Autodesk Inventor part; units mm, degrees
ref_plane "YZ Plane" through (0, 0, 0) normal (1, 0, 0) x (0, 1, 0)
ref_plane "XZ Plane" through (0, 0, 0) normal (0, 1, 0) x (-1, 0, 0)
ref_plane "XY Plane" through (0, 0, 0) normal (0, 0, 1) x (1, 0, 0)
sketch "Boceto1" plane through (0, 0, 0) normal (0, 0, 1) x (1, 0, 0)
  circle A0 centre (0, 0) radius 4
  circle A1 centre (0, 0) radius 1.5
  line L0 (0, -1) -> (1.5, -1)
  line L1 (1.5, -1) -> (-2.7531, -1)
  point P0 (1, -1.118)
  point P1 (1, 1.118)
  point P2 (-1.118, -1)
  point P3 (1.118, -1)
  dimension "d0" = 8
extrude "Extrusión1" add sketch "Boceto1" along normal blind 8 contours A0 | L1 L0 A1 picked at (-0.6553, -1.0791)
sketch "Boceto2" plane through (0, 0, 8) normal (0, 0, 1) x (1, 0, 0)
  circle A0 centre (0, 0) radius 8
  dimension "d3" = 16
extrude "Extrusión2" add sketch "Boceto2" along normal blind 10
sketch "Boceto3" plane through (0, 0, 18) normal (0, 0, 1) x (1, 0, 0)
  circle A0 centre (0, 0) radius 8
hole "Agujero1" at (0, 0, 18) direction (0, 0, -1) diameter 8 depth 8
sketch "Boceto5" plane through (0, 0, 0) normal (0, 1, 0) x (-1, 0, 0)
  line L0 (0, 0) -> (0, 4)
  circle A0 centre (0, 4) radius 1
  line L1 (0, 4) -> (0, 8)
  line L2 (0, 8) -> (0, 13)
  circle A1 centre (0, 13) radius 1.5
  dimension "d20" = 4
  dimension "d21" = 2
  dimension "d29" = 5
  dimension "d30" = 3
hole "Agujero3" at (0, 0, 4) direction (0, -1, 0) diameter 2 end through all
sketch "Boceto6" plane through (0, 0, 0) normal (0, 1, 0) x (-1, 0, 0)
  line L0 (0, 0) -> (0, 13)
  circle A0 centre (0, 13) radius 1.5
  dimension "d31" = 13
  dimension "d32" = 3
hole "Agujero4" at (0, 0, 13) direction (0, -1, 0) diameter 3 end through all
ref_plane "Plano de trabajo2" through (0, 0, 7) normal (0, 0, 1) x (-1, 0, 0)
sketch "Boceto7" plane through (0, 0, 7) normal (0, 0, 1) x (-1, 0, 0)
  circle A0 centre (0, 0) radius 17.5
  dimension "d42" = 35
extrude "Extrusión3" add sketch "Boceto7" along normal mid plane 1.5
sketch "Boceto8" plane through (0, 0, 7.75) normal (0, 0, 1) x (1, 0, 0)
  circle A0 centre (0, 0) radius 8
  circle A1 centre (0, 0) radius 17.5
  arc A2 (8.6603, -5) -> (10, 0) centre (0, 0) ccw
  arc A3 (14.2894, -8.25) -> (16.5, 0) centre (0, 0) ccw
  line L0 (10, 0) -> (16.5, 0)
  line L1 (0, 0) -> (16.5, 0) construction
  line L2 (8.6603, -5) -> (14.2894, -8.25)
  arc A4 (8.6603, 5) -> (5, 8.6603) centre (0, 0) ccw
  line L3 (8.6603, 5) -> (14.2894, 8.25)
  arc A5 (14.2894, 8.25) -> (8.25, 14.2894) centre (0, 0) ccw
  line L4 (5, 8.6603) -> (8.25, 14.2894)
  arc A6 (0, 10) -> (-5, 8.6603) centre (0, 0) ccw
  line L5 (0, 10) -> (0, 16.5)
  arc A7 (0, 16.5) -> (-8.25, 14.2894) centre (0, 0) ccw
  line L6 (-5, 8.6603) -> (-8.25, 14.2894)
  arc A8 (-8.6603, 5) -> (-10, 0) centre (0, 0) ccw
  line L7 (-8.6603, 5) -> (-14.2894, 8.25)
  arc A9 (-14.2894, 8.25) -> (-16.5, 0) centre (0, 0) ccw
  line L8 (-10, 0) -> (-16.5, 0)
  arc A10 (-8.6603, -5) -> (-5, -8.6603) centre (0, 0) ccw
  line L9 (-8.6603, -5) -> (-14.2894, -8.25)
  arc A11 (-14.2894, -8.25) -> (-8.25, -14.2894) centre (0, 0) ccw
  line L10 (-5, -8.6603) -> (-8.25, -14.2894)
  arc A12 (0, -10) -> (5, -8.6603) centre (0, 0) ccw
  line L11 (0, -10) -> (0, -16.5)
  arc A13 (0, -16.5) -> (8.25, -14.2894) centre (0, 0) ccw
  line L12 (5, -8.6603) -> (8.25, -14.2894)
  point P0 (0, 0)
  dimension "d45" = 2
  dimension "d46" = 1
  dimension "d50" = 360
extrude "Extrusión4" cut sketch "Boceto8" against normal through all contours A2 L0 A3 L2 | A4 L4 A5 L3 | A6 L6 A7 L5 | A8 L8 A9 L7 | A10 L10 A11 L9 | A12 L12 A13 L11
sketch "Boceto9" plane through (0, 0, 0) normal (0, 0, -1) x (-1, 0, 0)
  circle A0 centre (0, 0) radius 1.75
  dimension "d54" = 3.5
extrude "Extrusión5" cut sketch "Boceto9" against normal blind 1.5
sketch "Boceto10" plane through (0, 0, 10) normal (0, 0, 1) x (1, 0, 0)
  arc A0 (1.118, -1) -> (-1.118, -1) centre (0, 0) ccw
  circle A1 centre (0, 0) radius 1.75
  line L0 (1.118, -1) -> (-1.118, -1)
  point P0 (-1.4361, -1)
  point P1 (-1.7451, -0.1303)
extrude "Extrusión6" cut sketch "Boceto10" against normal blind 10 contours L0 A0
fillet "Empalme3" radius 2 1 edges at (-4, 0, 6.25)
properties part number "Acople"
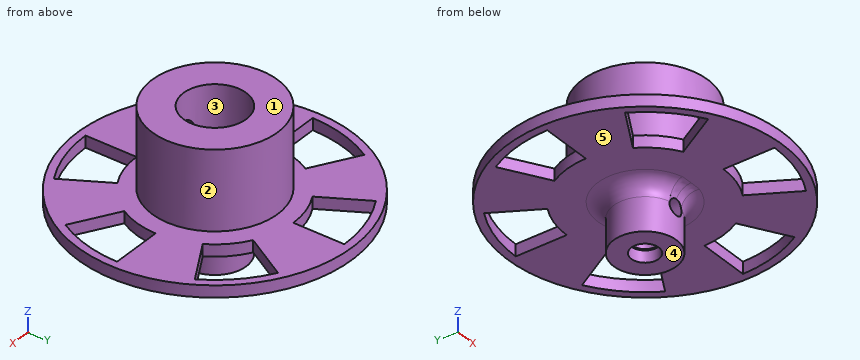
Input: part model. Units: mm. Frame: model coordinates. Face numbers are marked on the shaded views. A direction names the side the tool comes from. Coordinates: 2 decimals unless noted, no trailing zeros. Order: outer loops, then holes, each group sorted by start corner. A loop starts at its lowest first (then second) coordinate and runs counter-clockwise, first axis right, second up.
1. Cut plane B-B, the plane z = 10.5. Return loops of the section in (x, y), plus the area to 3 significant figures.
Checked values:
outline: circle Ø16 at (0, 0); hole circle Ø8 at (0, 0)
area: 151 mm2
2. Cut plane A-A, the plane x = 15. Return loops of the section in (y, z), plus the area to 3 significant figures.
Checked values:
outline: (-9.01, 6.25) - (-6.87, 6.25) - (-6.87, 7.75) - (-9.01, 7.75) - close; (0, 6.25) - (9.01, 6.25) - (9.01, 7.75) - (0, 7.75) - close
area: 16.7 mm2
3. Contact query for flat-ended pins moving along their axis: P1, Ø0.8, axis at x = 0.5, y = 0, coming from the -Z side; P2, Ø4, axis at x = 0.5, y = 0.5, coming from the +Z side; P3, Ø1.2, axis at x = -14, z = 7, coming from the +Y side; P4, Ø5, axis at x = 5, z = 13, coming from the +Y side. Output: stop coordinate, or through.
Checked values:
P1: passes through
P2: stops at z = 10
P3: stops at y = 11.26
P4: stops at y = 7.6
4. Ray query, line 1 along Y through (x, z) = (0, 1.1); line 2 along Y through (x, z) = (0, 9.55); line 3 along Z through (x, y) = (-5.5, 9). Return the intervals inside material, ascending.
Checked values:
line 1: y = -4 to -1.75, 1.75 to 4
line 2: y = -8 to -1, 1.5 to 8
line 3: z = 6.25 to 7.75
5. Cut plane D-D, the plane x = 4.5. Count the separate pieces of the cut face and the enclosed holes in it, plus the area to 3 significant figures.
Checked values:
separate pieces: 3
enclosed holes: 0
area: 175 mm2
6. Access query for the marked faces 4 and 5. Directions: +Z, -Z, +X, -X, +Y, -Y. A direction counts if a zero-diameter tool reaches every point of the face in a straight line with its end or side. Return the directions, or none.
Checked values:
face 4: -Z, +X, -X, +Y, -Y
face 5: -Z
7. Draft query along X for the marked faces 1, 2 and 3. Return one class per face: +X half, -X half, draft (parallel to the pull), parting line (faces both ways), or undercut.
Checked values:
face 1: draft
face 2: parting line
face 3: undercut
